Design review of the part built by this model. Coordinates are the model's own, in mm. A direction names the side the tool comes from. Coordinates: 2 decimals unless noted, no trailing zeros. Order: outer loops, then holes, each group sorted by start corner. A loop starts at its lowest first (then second) coordinate and runs counter-clockwise, first axis right, second up. Notation, with made-up numbers: (12.5, 1) -> (26.5, 1) arc R31 ccw to (26.5, 26) -> close; hole circle Ø9 at (79.25, 64.5). An arc over 180 degrees is marked (long way). Write item = value, one per line.
```python
from build123d import *

# Parameters (mm, degrees)
F0_W     = 55
F0_H     = 55
F0_W_2   = 45
F0_H_2   = 45
F1_DEPTH = 30
F2_W     = 15
F2_H     = 10
F3_DEPTH = 25


# Not quite as in the source:
# - a feature names something its author has since deleted; it is built from what else it names


with BuildPart() as f1:
    # F0 (on Front) → F1 (new body)
    with BuildSketch(Plane.XZ):
        Rectangle(F0_W, F0_H)
        Rectangle(F0_W_2, F0_H_2, mode=Mode.SUBTRACT)
    extrude(amount=F1_DEPTH)

    # F2 (on face) → F3 (cut)
    with BuildSketch(Plane.XY.offset(27.5)):
        with Locations((-2.9486052878, -12.4806062132)):
            Rectangle(F2_W, F2_H)
    extrude(amount=-F3_DEPTH, mode=Mode.SUBTRACT)


solid = f1.part
```
(1) Insertion check: pin 1 (4 mm diameter, centred on x = -5, z = 26, fed in from +Y); pin 2 (8 mm diameter, centred on x = -4.5, z = -15.5, fed in from -Y). Each pin has a flat end and moves straight along its axis. Give the tip position at first contact, or say it passes through.
Report:
pin_1 = 0
pin_2 = through
(2) For faces 1 (the flat face through (0, -18, 27.5)), 2 (the flat face through (-22.5, -15, 0)), 3 (the flat face through (-10.449, -13, 25)), list the 3-axis set-ups (+Z, -Z, +X, -X, +Y, -Y) from which the entire face can be reached by the end or side of a thin tool; tool diameter is ignored.
Report:
face_1 = +Z, +X, -X, +Y, -Y
face_2 = +Y, -Y
face_3 = +Z
(3) We need section D-D (y = -16.75). Write out the cut boundary in (x, z).
Report:
outline = (-27.5, -27.5) -> (27.5, -27.5) -> (27.5, 27.5) -> (4.55, 27.5) -> (4.55, 22.5) -> (22.5, 22.5) -> (22.5, -22.5) -> (-22.5, -22.5) -> (-22.5, 22.5) -> (-10.45, 22.5) -> (-10.45, 27.5) -> (-27.5, 27.5) -> close
(4) The part is to be moulded in two halves that separate along Z. For faces 4 (the flat face through (22.5, -15, 0)), 5 (the flat face through (-3, -7.481, 25)), 6 (the flat face through (0, -15, -22.5)), 7 (the flat face through (0, -15, -27.5)), say which applies: released by +Z, released by -Z, zero draft, split by the parting line, or undercut.
Report:
face_4 = undercut
face_5 = zero draft
face_6 = undercut
face_7 = released by -Z
(5) We need section C-C (x = -14). Write out the cut boundary in (y, z), and give its area (3 significant figures).
Report:
outline = (-30, -27.5) -> (0, -27.5) -> (0, -22.5) -> (-30, -22.5) -> close; (-30, 22.5) -> (0, 22.5) -> (0, 27.5) -> (-30, 27.5) -> close
area = 300 mm²
(6) For L1, parallel to X at y = -2.5, z = -5; L2, parallel to Z at x = 3.5, y = -13.25, list the stretches that pass through material, from the lowest coordinate up.
Report:
L1 = -27.5 to -22.5, 22.5 to 27.5
L2 = -27.5 to -22.5
(7) We need section A-A (z = 5). Write out the cut boundary in (x, y), and give its area (3 significant figures).
Report:
outline = (-27.5, -30) -> (-22.5, -30) -> (-22.5, 0) -> (-27.5, 0) -> close; (22.5, -30) -> (27.5, -30) -> (27.5, 0) -> (22.5, 0) -> close
area = 300 mm²
(8) We need section B-B (x = -5.5). Write out the cut boundary in (y, z), and give its area (3 significant figures).
Report:
outline = (-30, -27.5) -> (0, -27.5) -> (0, -22.5) -> (-30, -22.5) -> close; (-30, 22.5) -> (-17.48, 22.5) -> (-17.48, 27.5) -> (-30, 27.5) -> close; (-7.48, 22.5) -> (0, 22.5) -> (0, 27.5) -> (-7.48, 27.5) -> close
area = 250 mm²
